Work out the finished part from the listing and answer in its coordinate system (mm). Face numbers are marked on the shaded views. Coordinates: 2 decimals unless noted, no trailing zeros. Order: outer loops, then holes, each group sorted by start corner. A loop starts at its lowest first (then second) coordinate and runs counter-clockwise, first axis right, second up. Notation, with made-up numbers: (60, 24) -> (94, 24) arc R28 cw to (94, 43) -> close; hole circle Ø5 at (3.5, 69). An arc over 180 degrees is marked (long way). Use one line per item in the form item = value.
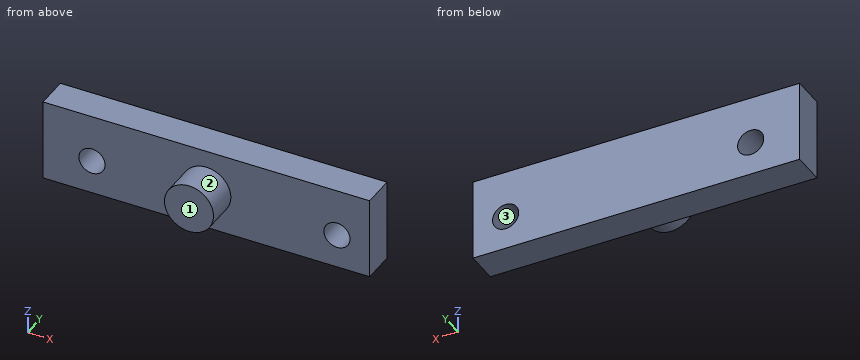
from build123d import *

# Parameters (mm, degrees)
SKETCH1_W           = 20
SKETCH1_H           = 5
SKETCH1_R           = 0.8
BOSS_EXTRUDE1_DEPTH = 2
SKETCH2_R           = 1.5
BOSS_EXTRUDE2_DEPTH = 2


with BuildPart() as part:
    # Sketch1 → Boss-Extrude1 (new body)
    with BuildSketch(Plane(origin=(0, 0, 0), x_dir=(1, 0, 0), z_dir=(0, 1, 0))):
        with Locations((9.677629379, 0.960024777)):
            Rectangle(SKETCH1_W, SKETCH1_H)
        with Locations((17.677629379, 1.377386897)):
            Circle(SKETCH1_R, mode=Mode.SUBTRACT)
        with Locations((2.677629379, 1.377386897)):
            Circle(SKETCH1_R, mode=Mode.SUBTRACT)
    extrude(amount=BOSS_EXTRUDE1_DEPTH)

    # Sketch2 → Boss-Extrude2 (add)
    with BuildSketch(Plane(origin=(0, 0, 0), x_dir=(-1, 0, 0), z_dir=(0, -1, 0))):
        with Locations((-9.677629379, 1.004049849)):
            Circle(SKETCH2_R)
    extrude(amount=BOSS_EXTRUDE2_DEPTH)


solid = part.part
(1) Section D-D on y = -1.4 is taken. Write down the section's boundary in (x, z).
Data:
outline = circle Ø3 at (9.68, -1)
(2) Section C-C on z = -0.1 is taken. Write down the section's boundary in (x, y), plus the area to 3 significant figures.
Data:
outline = (-0.32, 0) -> (8.48, 0) -> (8.48, -2) -> (10.87, -2) -> (10.87, 0) -> (19.68, 0) -> (19.68, 2) -> (-0.32, 2) -> close
area = 44.8 mm²
(3) Section A-A on x = 9 is taken. Write down the section's boundary in (y, z), plus the area to 3 significant figures.
Data:
outline = (-2, -2.34) -> (0, -2.34) -> (0, -3.46) -> (2, -3.46) -> (2, 1.54) -> (0, 1.54) -> (0, 0.33) -> (-2, 0.33) -> close
area = 15.4 mm²
(4) Section B-B on y = 1.45 is taken. Write down the section's boundary in (x, z), plus the area to 3 significant figures.
Data:
outline = (-0.32, -3.46) -> (19.68, -3.46) -> (19.68, 1.54) -> (-0.32, 1.54) -> close; hole circle Ø1.6 at (2.68, -1.38); hole circle Ø1.6 at (17.68, -1.38)
area = 96.0 mm²
(5) The mould has two halves that part along X. Classify the marked faces 1, 2 and 3: released by +X, released by -X, zero draft, split by the parting line, or undercut.
Data:
face_1 = zero draft
face_2 = split by the parting line
face_3 = undercut
(6) Straight lines are drawn through the part: line 1 along Z through (x, y) = (2.75, 1.4); line 2 along Y through (x, z) = (14, -0.45); line 3 along Z through (x, y) = (3, 0.05). For each, find the intervals that lie inside material, in ascending order.
Data:
line_1 = -3.46 to -2.17, -0.58 to 1.54
line_2 = 0 to 2
line_3 = -3.46 to -2.11, -0.65 to 1.54
